Part print with two shaded views. Sizes in mm from the minimum x, y, z corner. A direction names the side the tool comes from. Give positions to 0.01 mm unless a question says otherwise; leave off trailing zeros. Order: outer loops, then holes, each group sorted by start corner. A loop starts at its lowest first (then second) coordinate and runs counter-clockwise, first axis right, second up.
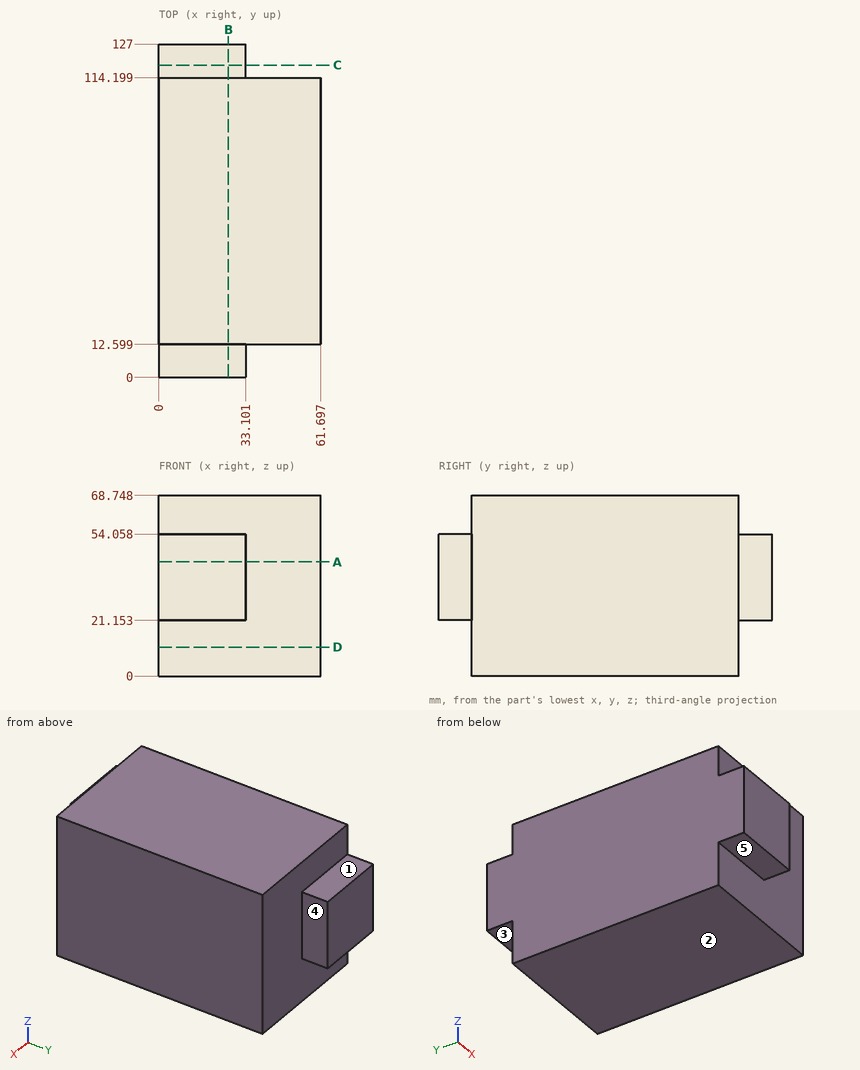
Item 1: Slice it at B-B (x = 26.5). Give the cut face in (y, z).
Item 2: Slice it at D-D (z = 11). Give the cut face in (x, y), and give its area (3 significant figures).
Item 3: Wall check: L1, parallel to Z at x = 19, y = 6; L2, parallel to Y at x = 38, z = 57. Give the ranges that are in metal, low to high.
Item 4: Tool access for the marked faces 1, 2, 3, 4 and 5: list every direction of +Z, -Z, +X, -X, +Y, -Y with a clear straight run to the whole face (end or side of a thin tool).
Item 5: Slice it at A-A (z = 43.5). Give the cut face in (x, y).
Item 6: Slice it at C-C (y = 119). Give the cut face in (x, z).
Item 7: Drop flat-ended pins along their axis: pin 1 Ø4 at (y, z) = (6, 41) entering from +X; pin 2 Ø3 at (x, z) = (27, 16) entering from -Y; pin 3 Ø10 at (x, y) = (11, 3.5) entering from +Z. Give the stop position or say it passes through.
A:
1. outline: (0, 21.15) - (12.6, 21.15) - (12.6, 0) - (114.2, 0) - (114.2, 21.15) - (127, 21.15) - (127, 54.06) - (114.2, 54.06) - (114.2, 68.75) - (12.6, 68.75) - (12.6, 54.06) - (0, 54.06) - close
2. outline: (0, 12.6) - (61.7, 12.6) - (61.7, 114.2) - (0, 114.2) - close
2. area: 6,270 mm2
3. L1: z = 21.15 to 54.06
3. L2: y = 12.6 to 114.2
4. face 1: +Z, +X, -X, +Y
4. face 2: -Z, +X, -X, +Y, -Y
4. face 3: -Z, +X, -X, +Y
4. face 4: +Z, -Z, +X, +Y
4. face 5: -Z, +X, -X, -Y
5. outline: (0, 0) - (33.1, 0) - (33.1, 12.6) - (61.7, 12.6) - (61.7, 114.2) - (33.1, 114.2) - (33.1, 127) - (0, 127) - close
6. outline: (0, 21.15) - (33.1, 21.15) - (33.1, 54.06) - (0, 54.06) - close
7. pin 1: stops at x = 33.1
7. pin 2: stops at y = 12.6
7. pin 3: stops at z = 54.06
